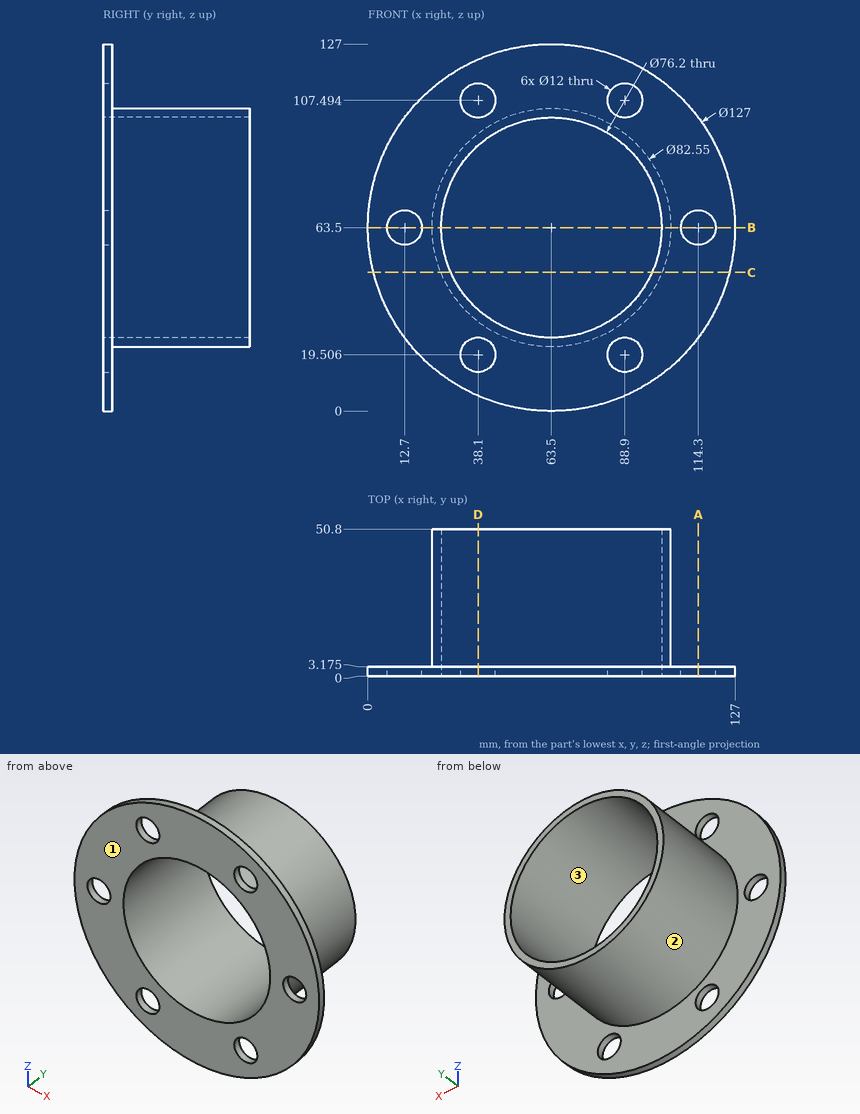
For this review, use the dimensioned drawing (mm, ordinates from the lowest corner) and the shaded views. Give positions to 0.01 mm unless a question says otherwise; leave off trailing zeros. Write each loop counter-clockwise with the first axis right and the second up, starting at its lowest first coordinate (ties: lowest second). Pieces come first, ordered by that corner, then holes. Notation, with made-up numbers: M -21,22 L -15,22 A11 ccw -15,35 Z; hole C -18,89.5 d4. An arc over 180 degrees is marked long. Answer as a JSON object with one key per item and string values. Group by question number.
1) We need section A-A (x = 114.3). Give the boundary of the cut face in (y, z) (3 decimals), and give its area (3 significant figures).
2) Clearance check with flat-ended pins moving along their axes: pin 1 Ø14 at (x, z) = (114.3, 63.5) entering from +Y (3 decimals); pin 2 Ø3 at (y, z) = (41.5, 40.5) entering from -X; pin 3 Ø6 at (x, y) = (49.5, 32.5) entering from +Z; pin 4 Ø7 at (x, z) = (88.9, 107.49) entering from +Y (3 decimals). State where each tip first meets the part, or that it passes through.
3) Mouldability with a two-part tool opening along X and no side actions: class the marked faces 1, 2 and 3 as released by +X, released by -X, zero draft, split by the parting line, or undercut.
4) For line 1 along X through (y, z) = (18.5, 63); line 2 along Y through (x, z) = (108, 35) (3 decimals); line 3 along Z through (x, y) = (12, 1), list the stretches that pass through material, from the lowest coordinate up.
5) We need section B-B (z = 63.5). Give the boundary of the cut face in (x, y) (3 decimals).
6) We need section D-D (x = 38.1). Give the boundary of the cut face in (y, z) (3 decimals).
7) We need section C-C (z = 48). Give the boundary of the cut face in (x, y) (1 decimal), and give its area (3 significant figures).
Answer key:
{
 "1": {"outline": "M 0,25.4 L 3.175,25.4 L 3.175,57.5 L 0,57.5 Z; M 0,69.5 L 3.175,69.5 L 3.175,101.6 L 0,101.6 Z", "area": "204 mm²"},
 "2": {"pin 1": "stops at y = 3.175", "pin 2": "stops at x = 28.27", "pin 3": "stops at z = 103.28", "pin 4": "passes through"},
 "3": {"face 1": "zero draft", "face 2": "split by the parting line", "face 3": "undercut"},
 "4": {"line 1": "x = 22.23 to 25.4, 101.6 to 104.77", "line 2": "y = 0 to 3.175", "line 3": "z = 26.35 to 57.54, 69.46 to 100.65"},
 "5": {"outline": "M 0,0 L 6.7,0 L 6.7,3.175 L 0,3.175 Z; M 18.7,0 L 25.4,0 L 25.4,50.8 L 22.225,50.8 L 22.225,3.175 L 18.7,3.175 Z; M 101.6,0 L 108.3,0 L 108.3,3.175 L 104.775,3.175 L 104.775,50.8 L 101.6,50.8 Z; M 120.3,0 L 127,0 L 127,3.175 L 120.3,3.175 Z"},
 "6": {"outline": "M 0,5.301 L 3.175,5.301 L 3.175,13.506 L 0,13.506 Z; M 0,25.506 L 3.175,25.506 L 3.175,30.966 L 50.8,30.966 L 50.8,35.102 L 0,35.102 Z; M 0,91.898 L 50.8,91.898 L 50.8,96.034 L 3.175,96.034 L 3.175,101.494 L 0,101.494 Z; M 0,113.494 L 3.175,113.494 L 3.175,121.699 L 0,121.699 Z"},
 "7": {"outline": "M 1.9,0 L 28.7,0 L 28.7,50.8 L 25.2,50.8 L 25.2,3.2 L 1.9,3.2 Z; M 98.3,0 L 125.1,0 L 125.1,3.2 L 101.8,3.2 L 101.8,50.8 L 98.3,50.8 Z", "area": "499 mm²"}
}
